Here's how the part is built. I have some questions about the finished solid (model axes, mm). Face numbers are marked on the shaded views. A direction names the side the tool comes from. Give positions to 0.01 mm unless a question says otherwise; leave off trailing zeros. Loops run counter-clockwise (first coordinate to the right, second up) from the corner with the lowest first, then second, coordinate; pieces in that order, holes last. Notation, with made-up numbers: M -27,78 L -5,78 A11 ccw -5,94 Z; hole C 77,64 d1. An arc over 180 degrees is marked long. Answer as CSV lines item,"result". Start each with the question number.
Item 1: For the marked faces 5 and 6, which set-ups out of +Z, -Z, +X, -X, +Y, -Y let a thin tool reach every point of the face, with its end or its side?
Item 2: I want a section at A-A on x = 20. List the corners of the cut face in (y, z) for me.
Item 3: Will these pins go through, and if not, where does the flat tip stop? P1, Ø4.5, axis at x = 23, z = -3.5, coming from the +Y side; P2, Ø8, axis at x = 17, z = 10.5, coming from the -Y side; P3, Ø1.6, axis at y = 18.5, z = -1, coming from the +X side; P4, Ø0.8, axis at y = 18.5, z = 0.5, coming from the -X side.
Item 4: I want a section at C-C on z = -6. List the corners of the cut face in (x, y) for me, plus the area to 3 significant figures.
Item 5: If we mould it in two halves opening along X, with no side actions, what happens to the marked faces 1, 2, 3 and 4? For each: released by +X, released by -X, zero draft, split by the parting line, or undercut.
Item 6: I want a section at B-B on y = 3.25. List the corners of the cut face in (x, z) for me.
Item 7: If I drill on line 1 along X through (y, z) = (4, 27); line 2 along Z through (x, y) = (3, 9); line 3 along Y through (x, z) = (3.5, -1.5), over which ranges is the centre line in solid material (lowest first)? Write a range as from..to.
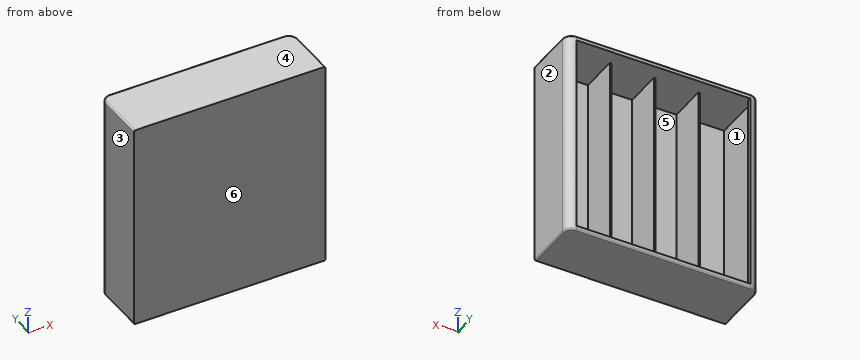
from build123d import *

# Parameters (mm, degrees)
SKETCH1_W           = 65
SKETCH1_H           = 70
BOSS_EXTRUDE1_DEPTH = 19.5
FILLET1_R           = 3
FILLET2_R           = 0.5
SHELL1_START        = -33.5
SHELL1_DEPTH        = 67
SKETCH2_W           = 0.5
SKETCH2_H           = 67
EXTRUDE_THIN1_DEPTH = 13
LPATTERN1_COUNT     = 2
LPATTERN1_PITCH     = 15
LPATTERN1_COL_COUNT = 2
LPATTERN1_COL_PITCH = 15


# Read off the part's stored shape, not the designer's step: Shell1
with BuildPart() as part:
    # Sketch1 → Boss-Extrude1 (new body)
    with BuildSketch(Plane(origin=(0, 0, 0), x_dir=(1, 0, 0), z_dir=(0, 1, 0))):
        Rectangle(SKETCH1_W, SKETCH1_H)
    extrude(amount=BOSS_EXTRUDE1_DEPTH)

    # Fillet1
    fillet1_edges = [part.edges().sort_by_distance(p)[0] for p in [
        (32.5, 19.5, 0),
        (-32.5, 19.5, 0),
    ]]
    fillet(fillet1_edges, radius=FILLET1_R)

    # Fillet2
    fillet2_edges = [part.edges().sort_by_distance(p)[0] for p in [
        (0, 19.5, 35),
        (0, 19.5, -35),
        (-32.5, 8.25, -35),
        (32.5, 8.25, -35),
        (-31.621320344, 18.621320344, -35),
        (31.621320344, 18.621320344, -35),
        (32.5, 8.25, 35),
        (-32.5, 8.25, 35),
        (-31.621320344, 18.621320344, 35),
        (31.621320344, 18.621320344, 35),
    ]]
    fillet(fillet2_edges, radius=FILLET2_R)

    # Shell1 outline → Shell1 (cut)
    with BuildSketch(Plane.XY.offset(SHELL1_START)):
        with BuildLine():
            Line((29.5, 18), (29.5, 19.5))
            Line((29.5, 19.5), (-29.5, 19.5))
            Line((-29.5, 19.5), (-29.5, 18))
            ThreePointArc((-29.5, 18), (-30.560660172, 17.560660172), (-31, 16.5))
            Line((-31, 16.5), (-31, 1.5))
            Line((-31, 1.5), (31, 1.5))
            Line((31, 1.5), (31, 16.5))
            ThreePointArc((31, 16.5), (30.560660172, 17.560660172), (29.5, 18))
        make_face()
    extrude(amount=SHELL1_DEPTH, mode=Mode.SUBTRACT)

    # Sketch2 → Extrude-Thin1 (add)
    with BuildSketch(Plane(origin=(0, 1.5, 0), x_dir=(1, 0, 0), z_dir=(0, 1, 0))):
        Rectangle(SKETCH2_W, SKETCH2_H)
    extrude_thin1 = extrude(amount=EXTRUDE_THIN1_DEPTH)

    # LPattern1: Extrude-Thin1 ×2
    with Locations(*[(-i * LPATTERN1_PITCH, 0, 0) for i in range(1, LPATTERN1_COUNT)]):
        add(extrude_thin1)

    # LPattern1 col: Extrude-Thin1 ×2
    with Locations(*[(i * LPATTERN1_COL_PITCH, 0, 0) for i in range(1, LPATTERN1_COL_COUNT)]):
        add(extrude_thin1)


solid = part.part
Result:
1,face 5,"+Y"
1,face 6,"+Z, -Z, +X, -X, -Y"
2,outline,"M 0,-35 L 19,-35 A0.5 ccw 19.5,-34.5 L 19.5,-33.5 L 1.5,-33.5 L 1.5,33.5 L 19.5,33.5 L 19.5,34.5 A0.5 ccw 19,35 L 0,35 Z"
3,P1,"y = 1.5"
3,P2,"y = 0"
3,P3,"x = 32.25"
3,P4,"x = -32.04"
4,outline,"M -32.5,0 L 32.5,0 L 32.5,16.5 A3 ccw 29.5,19.5 L 29.5,18 A1.5 cw 31,16.5 L 31,1.5 L 15.25,1.5 L 15.25,14.5 L 14.75,14.5 L 14.75,1.5 L 0.25,1.5 L 0.25,14.5 L -0.25,14.5 L -0.25,1.5 L -14.75,1.5 L -14.75,14.5 L -15.25,14.5 L -15.25,1.5 L -31,1.5 L -31,16.5 A1.5 cw -29.5,18 L -29.5,19.5 A3 ccw -32.5,16.5 Z"
4,area,"173 mm^2"
5,face 1,"undercut"
5,face 2,"released by +X"
5,face 3,"released by -X"
5,face 4,"zero draft"
6,outline,"M -32.5,-34.5 A0.5 ccw -32,-35 L 32,-35 A0.5 ccw 32.5,-34.5 L 32.5,34.5 A0.5 ccw 32,35 L -32,35 A0.5 ccw -32.5,34.5 Z; hole M -31,-33.5 L -15.25,-33.5 L -15.25,33.5 L -31,33.5 Z; hole M -14.75,-33.5 L -0.25,-33.5 L -0.25,33.5 L -14.75,33.5 Z; hole M 0.25,-33.5 L 14.75,-33.5 L 14.75,33.5 L 0.25,33.5 Z; hole M 15.25,-33.5 L 31,-33.5 L 31,33.5 L 15.25,33.5 Z"
7,line 1,"-32.5..-31, -15.25..-14.75, -0.25..0.25, 14.75..15.25, 31..32.5"
7,line 2,"-35..-33.5, 33.5..35"
7,line 3,"0..1.5"
